Design review of the part built by this model. Coordinates are the model's own, in mm. A direction names the side the tool comes from. Round coordinates to 2 decimals unless told otherwise and drop trailing zeros. Order: outer loops, then holes, each group sorted by start corner. A loop starts at its lowest first (then second) coordinate and runs counter-clockwise, first axis right, second up. Notation, with made-up numbers: (68.25, -0.75) - (116.25, -0.75) arc R19 ccw to (116.25, 16.25) - close; hole circle Ø10 at (38.5, 56.25). An arc over 180 degrees is marked (long way). Write item = value, one per line.
from build123d import *

# Parameters (mm, degrees)
SKETCH1_W           = 150
SKETCH1_H           = 250
BOSS_EXTRUDE1_DEPTH = 6.35
SKETCH2_R           = 1.5875
SKETCH2_W           = 80.264
SKETCH2_H           = 12.954
CUT_EXTRUDE1_DEPTH  = 196.359469952
SKETCH3_R           = 3
CUT_EXTRUDE2_DEPTH  = 196.359469952
FILLET1_R           = 5


with BuildPart() as part:
    # Sketch1 → Boss-Extrude1 (new body)
    with BuildSketch(Plane(origin=(0, 0, 0), x_dir=(1, 0, 0), z_dir=(0, 1, 0))):
        with Locations((75, 0)):
            Rectangle(SKETCH1_W, SKETCH1_H)
    extrude(amount=-BOSS_EXTRUDE1_DEPTH)

    # Sketch2 → Cut-Extrude1 (cut, through all)
    with BuildSketch(Plane(origin=(0, 0, 0), x_dir=(1, 0, 0), z_dir=(0, 1, 0))):
        with Locations(Location((59.125, -80.424, 0), (0, 0, 270))):
            Circle(SKETCH2_R)
        with Locations(Location((59.125, -74.074, 0), (0, 0, 270))):
            Circle(SKETCH2_R)
        with Locations(Location((59.125, -67.724, 0), (0, 0, 270))):
            Circle(SKETCH2_R)
        with Locations(Location((59.125, -61.374, 0), (0, 0, 270))):
            Circle(SKETCH2_R)
        with Locations(Location((59.125, -55.024, 0), (0, 0, 270))):
            Circle(SKETCH2_R)
        with Locations(Location((59.125, -48.674, 0), (0, 0, 270))):
            Circle(SKETCH2_R)
        with Locations(Location((59.125, -42.324, 0), (0, 0, 270))):
            Circle(SKETCH2_R)
        with Locations(Location((90.875, -80.424, 0), (0, 0, 270))):
            Circle(SKETCH2_R)
        with Locations(Location((90.875, -74.074, 0), (0, 0, 270))):
            Circle(SKETCH2_R)
        with Locations(Location((90.875, -67.724, 0), (0, 0, 270))):
            Circle(SKETCH2_R)
        with Locations(Location((90.875, -61.374, 0), (0, 0, 270))):
            Circle(SKETCH2_R)
        with Locations(Location((90.875, -55.024, 0), (0, 0, 270))):
            Circle(SKETCH2_R)
        with Locations(Location((90.875, -48.674, 0), (0, 0, 270))):
            Circle(SKETCH2_R)
        with Locations(Location((90.875, -42.324, 0), (0, 0, 270))):
            Circle(SKETCH2_R)
        with Locations(Location((59.125, 80.424, 0), (0, 0, 270))):
            Circle(SKETCH2_R)
        with Locations(Location((59.125, 74.074, 0), (0, 0, 270))):
            Circle(SKETCH2_R)
        with Locations(Location((59.125, 67.724, 0), (0, 0, 270))):
            Circle(SKETCH2_R)
        with Locations(Location((59.125, 61.374, 0), (0, 0, 270))):
            Circle(SKETCH2_R)
        with Locations(Location((59.125, 55.024, 0), (0, 0, 270))):
            Circle(SKETCH2_R)
        with Locations(Location((59.125, 48.674, 0), (0, 0, 270))):
            Circle(SKETCH2_R)
        with Locations(Location((59.125, 42.324, 0), (0, 0, 270))):
            Circle(SKETCH2_R)
        with Locations(Location((90.875, 80.424, 0), (0, 0, 270))):
            Circle(SKETCH2_R)
        with Locations(Location((90.875, 74.074, 0), (0, 0, 270))):
            Circle(SKETCH2_R)
        with Locations(Location((90.875, 67.724, 0), (0, 0, 270))):
            Circle(SKETCH2_R)
        with Locations(Location((90.875, 61.374, 0), (0, 0, 270))):
            Circle(SKETCH2_R)
        with Locations(Location((90.875, 55.024, 0), (0, 0, 270))):
            Circle(SKETCH2_R)
        with Locations(Location((90.875, 48.674, 0), (0, 0, 270))):
            Circle(SKETCH2_R)
        with Locations(Location((90.875, 42.324, 0), (0, 0, 270))):
            Circle(SKETCH2_R)
        with Locations((75, -110.523)):
            Rectangle(SKETCH2_W, SKETCH2_H)
        with Locations((75, 110.523)):
            Rectangle(SKETCH2_W, SKETCH2_H)
    extrude(amount=-CUT_EXTRUDE1_DEPTH, mode=Mode.SUBTRACT)

    # Sketch3 → Cut-Extrude2 (cut, through all)
    with BuildSketch(Plane(origin=(0, 0, 0), x_dir=(1, 0, 0), z_dir=(0, 1, 0))):
        with Locations(Location((25, -14.975, 0), (0, 0, 270))):
            Circle(SKETCH3_R)
        with Locations(Location((25, -34.475, 0), (0, 0, 270))):
            Circle(SKETCH3_R)
        with Locations(Location((25, 14.975, 0), (0, 0, 270))):
            Circle(SKETCH3_R)
        with Locations(Location((25, 34.475, 0), (0, 0, 270))):
            Circle(SKETCH3_R)
        with Locations(Location((125, -14.975, 0), (0, 0, 270))):
            Circle(SKETCH3_R)
        with Locations(Location((125, -34.475, 0), (0, 0, 270))):
            Circle(SKETCH3_R)
        with Locations(Location((125, 14.975, 0), (0, 0, 270))):
            Circle(SKETCH3_R)
        with Locations(Location((125, 34.475, 0), (0, 0, 270))):
            Circle(SKETCH3_R)
    extrude(amount=-CUT_EXTRUDE2_DEPTH, mode=Mode.SUBTRACT)

    # Fillet1
    fillet1_edges = [part.edges().sort_by_distance(p)[0] for p in [
        (0, -3.175, -125),
        (150, -3.175, -125),
        (150, -3.175, 125),
        (0, -3.175, 125),
    ]]
    fillet(fillet1_edges, radius=FILLET1_R)


solid = part.part
Item 1: For line 1 along Z through (x, y) = (76, -1); line 2 along X through (y, z) = (-2.75, -34); line 3 along X through (y, z) = (-3.25, -32), list the stretches that pass through material, from the lowest coordinate up. Write a range as [from, to].
Data:
line_1 = [-125, -117], [-104.05, 104.05], [117, 125]
line_2 = [0, 22.04], [27.96, 122.04], [127.96, 150]
line_3 = [0, 23.3], [26.7, 123.3], [126.7, 150]
Item 2: Take a section at A-A, the plane x = 79. State the section outline as (y, z) points, and give its area (3 significant figures).
Data:
outline = (-6.35, -125) - (0, -125) - (0, -117) - (-6.35, -117) - close; (-6.35, -104.05) - (0, -104.05) - (0, 104.05) - (-6.35, 104.05) - close; (-6.35, 117) - (0, 117) - (0, 125) - (-6.35, 125) - close
area = 1,420 mm2
Item 3: For faces 1 (the face through (34.868, -3, 111)), 2 (the face through (74, -3, 125)), list the 3-axis set-ups (+Z, -Z, +X, -X, +Y, -Y) from which the entire face can be reached by the end or side of a thin tool; tool diameter is ignored.
Data:
face_1 = +Y, -Y
face_2 = +Z, +X, -X, +Y, -Y
Item 4: Insertion check: P1, Ø3, axis at x = 90.875, z = -80.424, coming from the +Y side. The pin has a flat end and moves straight along its axis. Give the tip position at first contact, or say it passes through.
Data:
P1 = through
Item 5: The part is to be moulded in two halves that separate along Z. For faces 3 (the face through (74, -3, -125)), 4 (the face through (34.868, -3, -110)), 5 (the face through (74, -6.35, -2)), say which applies: +Z half, -Z half, draft (parallel to the pull), parting line (faces both ways), or undercut.
Data:
face_3 = -Z half
face_4 = undercut
face_5 = draft
Item 6: Take a section at B-B, the plane x = 25. State the section outline as (y, z) points (3 decimals), and give its area (3 significant figures).
Data:
outline = (-6.35, -125) - (0, -125) - (0, -37.475) - (-6.35, -37.475) - close; (-6.35, -31.475) - (0, -31.475) - (0, -17.975) - (-6.35, -17.975) - close; (-6.35, -11.975) - (0, -11.975) - (0, 11.975) - (-6.35, 11.975) - close; (-6.35, 17.975) - (0, 17.975) - (0, 31.475) - (-6.35, 31.475) - close; (-6.35, 37.475) - (0, 37.475) - (0, 125) - (-6.35, 125) - close
area = 1,440 mm2
Item 7: Take a section at C-C, the plane y = -1.25. Count the separate pieces of the cut face and the enclosed holes in it, and give its area (3 significant figures).
Data:
separate_pieces = 1
enclosed_holes = 38
area = 35,000 mm2
